Model file for the job. Use its own axes, mm. A direction names the side the tool comes from. Round coordinates to 2 decimals unless told otherwise and drop trailing zeros. Order: outer loops, then holes, each group sorted by start corner. A loop starts at its lowest first (then second) coordinate and runs counter-clockwise, first axis right, second up. Notation, with made-up numbers: (23.25, -28) - (51.25, -28) arc R23 cw to (51.25, -1) - close; hole circle Ø4 at (-40, -36.75). An arc over 180 degrees is marked (long way). Use one line per item in the form item = value.
from build123d import *

# Parameters (mm, degrees)
SKETCH_1_R          = 41
SKETCH_1_R_2        = 1.7
EXTRUDE_1_DEPTH     = 30
FILLET_1_R          = 3
SKETCH_2_R          = 3
CUT_EXTRUDE_1_DEPTH = 3
DRAFT_1_ANGLE       = -2
FILLET_4_R          = 1


with BuildPart() as part:
    # 草图1 → 凸台-拉伸1 (new body)
    with BuildSketch(Plane(origin=(0, 0, 0), x_dir=(1, 0, 0), z_dir=(0, 1, 0))):
        with BuildLine():
            ThreePointArc((45.836734694, 3.872176727), (32.526911935, 32.526911935), (3.872176727, 45.836734694))
            ThreePointArc((3.872176727, 45.836734694), (0, 54), (-3.872176727, 45.836734694))
            ThreePointArc((-3.872176727, 45.836734694), (-32.526911935, 32.526911935), (-45.836734694, 3.872176727))
            ThreePointArc((-45.836734694, 3.872176727), (-54, 0), (-45.836734694, -3.872176727))
            ThreePointArc((-45.836734694, -3.872176727), (-32.526911935, -32.526911935), (-3.872176727, -45.836734694))
            ThreePointArc((-3.872176727, -45.836734694), (0, -54), (3.872176727, -45.836734694))
            ThreePointArc((3.872176727, -45.836734694), (32.526911935, -32.526911935), (45.836734694, -3.872176727))
            ThreePointArc((45.836734694, -3.872176727), (54, 0), (45.836734694, 3.872176727))
        make_face()
        with Locations(Location((0, 0, 0), (0, 0, 270))):
            Circle(SKETCH_1_R, mode=Mode.SUBTRACT)
        with Locations(Location((0, 49, 0), (0, 0, 270))):
            Circle(SKETCH_1_R_2, mode=Mode.SUBTRACT)
        with Locations(Location((49, 0, 0), (0, 0, 270))):
            Circle(SKETCH_1_R_2, mode=Mode.SUBTRACT)
        with Locations(Location((0, -49, 0), (0, 0, 270))):
            Circle(SKETCH_1_R_2, mode=Mode.SUBTRACT)
        with Locations(Location((-49, 0, 0), (0, 0, 270))):
            Circle(SKETCH_1_R_2, mode=Mode.SUBTRACT)
    extrude(amount=EXTRUDE_1_DEPTH)

    # 圆角1
    fillet_1_edges = [part.edges().sort_by_distance(p)[0] for p in [
        (-45.836734694, 15, 3.872176727),
        (-45.836734694, 15, -3.872176727),
        (-3.872176727, 15, -45.836734694),
        (3.872176727, 15, -45.836734694),
        (45.836734694, 15, -3.872176727),
        (45.836734694, 15, 3.872176727),
        (3.872176727, 15, 45.836734694),
        (-3.872176727, 15, 45.836734694),
    ]]
    fillet(fillet_1_edges, radius=FILLET_1_R)

    # 草图2 → 切除-拉伸1 (cut)
    with BuildSketch(Plane(origin=(0, 30, 0), x_dir=(1, 0, 0), z_dir=(0, 1, 0))):
        with Locations(Location((0, 49, 0), (0, 0, 270))):
            Circle(SKETCH_2_R)
        with Locations(Location((-49, 0, 0), (0, 0, 270))):
            Circle(SKETCH_2_R)
        with Locations(Location((0, -49, 0), (0, 0, 270))):
            Circle(SKETCH_2_R)
        with Locations(Location((49, 0, 0), (0, 0, 270))):
            Circle(SKETCH_2_R)
    extrude(amount=-CUT_EXTRUDE_1_DEPTH, mode=Mode.SUBTRACT)

    # 拔模1
    draft_1_faces = [part.faces().sort_by_distance(p)[0] for p in [
        (0, 15, -41),
    ]]
    draft(draft_1_faces, Plane(origin=(0, 0, 24.5), x_dir=(0, 0, -1), z_dir=(0, -1, 0)), DRAFT_1_ANGLE)

    # 圆角4
    fillet_4_edges = [part.edges().sort_by_distance(p)[0] for p in [
        (0, 30, -42.047623085),
    ]]
    fillet(fillet_4_edges, radius=FILLET_4_R)


solid = part.part
(1) Slice it at A-A on x = 0. Give the cut face in (y, z).
Report:
outline = (0, -54) - (30, -54) - (30, -52) - (27, -52) - (27, -50.7) - (0, -50.7) - close; (0, -47.3) - (27, -47.3) - (27, -46) - (30, -46) - (30, -43.01) arc R1 ccw to (29.03, -42.01) - (0, -41) - close; (0, 41) - (29.03, 42.01) arc R1 ccw to (30, 43.01) - (30, 46) - (27, 46) - (27, 47.3) - (0, 47.3) - close; (0, 50.7) - (27, 50.7) - (27, 52) - (30, 52) - (30, 54) - (0, 54) - close
(2) Slice it at B-B on z = 0. Give the cut face in (x, y).
Report:
outline = (-54, 0) - (-50.7, 0) - (-50.7, 27) - (-52, 27) - (-52, 30) - (-54, 30) - close; (-47.3, 0) - (-41, 0) - (-42.01, 29.03) arc R1 ccw to (-43.01, 30) - (-46, 30) - (-46, 27) - (-47.3, 27) - close; (41, 0) - (47.3, 0) - (47.3, 27) - (46, 27) - (46, 30) - (43.01, 30) arc R1 ccw to (42.01, 29.03) - close; (50.7, 0) - (54, 0) - (54, 30) - (52, 30) - (52, 27) - (50.7, 27) - close
(3) Pull direction X, two halves, no side cores. Call faces 1 (the face through (-24, 30, -36)), 2 (the face through (32.81, 14.79, -32.24)), 3 (the face through (-46, 29, 0)): released by +X, released by -X, zero draft, split by the parting line, or undercut.
Report:
face_1 = zero draft
face_2 = released by +X
face_3 = undercut
(4) Probe probe 1 along X at (y, z) = (29.35, 0); probe 2 along Z at (x, y) = (0, 8); probe 3 along X at (y, z) = (5, -1.5). List the from-to ranges inside material, lowest first. Write a range as [from, to].
Report:
probe_1 = [-54, -52], [-46, -42.08], [42.08, 46], [52, 54]
probe_2 = [-54, -50.7], [-47.3, -41.28], [41.28, 47.3], [50.7, 54]
probe_3 = [-53.77, -49.8], [-48.2, -41.15], [41.15, 48.2], [49.8, 53.77]
(5) Tool access for faces 4 (the face through (0.07, 13.31, 47.3)), 5 (the face through (0, 29, 46)): list every direction of +Z, -Z, +X, -X, +Y, -Y with a clear straight run to the whole face (end or side of a thin tool).
Report:
face_4 = +Y, -Y
face_5 = +Y
(6) Slice it at C-C on y = 21. Count the separate pieces of the cut face and the enclosed holes in it, then the cut area to 3 significant figures.
Report:
separate_pieces = 1
enclosed_holes = 5
area = 1,430 mm2
(7) Pin check, flat tips, straight feed: pin 1 (3.5 mm diameter, centred on x = 0, z = 49, fed in from -Y); pin 2 (5 mm diameter, centred on x = -49, z = 0, fed in from +Y); pin 3 (3 mm diameter, centred on x = 32.5, y = 8, fed in from +Z); pin 4 (4 mm diameter, centred on y = 21, z = 28.5, fed in from +X). Stop position of each tip, or through.
Report:
pin_1 = 0
pin_2 = 27
pin_3 = 33.99
pin_4 = 37.6
